from build123d import *

# Parameters (mm, degrees)
SKETCH3_W            = 2.76715
SKETCH3_H            = 2.76715
BOSS_EXTRUDE1_DEPTH  = 5
SKETCH4_W            = 2.76715
SKETCH4_H            = 2.76715
BOSS_EXTRUDE2_DEPTH  = 7.5
SKETCH5_W            = 2.76715
SKETCH5_H            = 2.76715
BOSS_EXTRUDE3_DEPTH  = 7.5
SKETCH6_W            = 2.76715
SKETCH6_H            = 2.76715
BOSS_EXTRUDE4_DEPTH  = 7.5
SKETCH7_W            = 2.76715
SKETCH7_H            = 2.76715
BOSS_EXTRUDE5_DEPTH  = 7.5
SKETCH8_W            = 2.76715
SKETCH8_H            = 2.76715
BOSS_EXTRUDE6_DEPTH  = 7.5
SKETCH9_W            = 2.76715
SKETCH9_H            = 2.76715
BOSS_EXTRUDE7_DEPTH  = 7.5
SKETCH10_W           = 2.76715
SKETCH10_H           = 2.76715
BOSS_EXTRUDE8_DEPTH  = 7.5
SKETCH11_W           = 2.76715
SKETCH11_H           = 2.76715
BOSS_EXTRUDE9_DEPTH  = 7.5
SKETCH12_W           = 2.76715
SKETCH12_H           = 2.76715
BOSS_EXTRUDE10_DEPTH = 7.5
SKETCH13_W           = 2.76715
SKETCH13_H           = 2.76715
BOSS_EXTRUDE11_DEPTH = 3.75
SKETCH14_W           = 2.76715
SKETCH14_H           = 2.76715
BOSS_EXTRUDE12_DEPTH = 10
SKETCH15_W           = 2.76715
SKETCH15_H           = 2.76715
BOSS_EXTRUDE13_DEPTH = 7.5
SKETCH16_W           = 2.76715
SKETCH16_H           = 2.76715
BOSS_EXTRUDE14_DEPTH = 3.75
SKETCH17_W           = 2.76715
SKETCH17_H           = 2.76715
BOSS_EXTRUDE15_DEPTH = 10
CUT_EXTRUDE3_START   = -0.5
CUT_EXTRUDE3_DEPTH   = 1.76715


with BuildPart() as part:
    # Sketch3 → Boss-Extrude1 (new, symmetric)
    with BuildSketch(Plane.XY):
        Rectangle(SKETCH3_W, SKETCH3_H)
    extrude(amount=BOSS_EXTRUDE1_DEPTH, both=True)

    # Sketch4 → Boss-Extrude2 (add)
    with BuildSketch(Plane(origin=(1.383575, 0, 0), x_dir=(0, 0, -1), z_dir=(1, 0, 0))):
        with Locations((-3.616425, 0)):
            Rectangle(SKETCH4_W, SKETCH4_H)
        with Locations((3.616425, 0)):
            Rectangle(SKETCH4_W, SKETCH4_H)
    extrude(amount=BOSS_EXTRUDE2_DEPTH)

    # Sketch5 → Boss-Extrude3 (add)
    with BuildSketch(Plane.XY.offset(5)):
        with Locations((7.5, 0)):
            Rectangle(SKETCH5_W, SKETCH5_H)
    extrude(amount=BOSS_EXTRUDE3_DEPTH)

    # Sketch6 → Boss-Extrude4 (add)
    with BuildSketch(Plane.ZY.offset(-6.116425)):
        with Locations((11.116425, 0)):
            Rectangle(SKETCH6_W, SKETCH6_H)
    extrude(amount=BOSS_EXTRUDE4_DEPTH)

    # Sketch7 → Boss-Extrude5 (add)
    with BuildSketch(Plane.XY.offset(12.5)):
        Rectangle(SKETCH7_W, SKETCH7_H)
    extrude(amount=BOSS_EXTRUDE5_DEPTH)

    # Sketch8 → Boss-Extrude6 (add)
    with BuildSketch(Plane(origin=(0, 0, -5), x_dir=(-1, 0, 0), z_dir=(0, 0, -1))):
        with Locations((-7.5, 0)):
            Rectangle(SKETCH8_W, SKETCH8_H)
    extrude(amount=BOSS_EXTRUDE6_DEPTH)

    # Sketch9 → Boss-Extrude7 (add)
    with BuildSketch(Plane.ZY.offset(-6.116425)):
        with Locations((-11.116425, 0)):
            Rectangle(SKETCH9_W, SKETCH9_H)
    extrude(amount=BOSS_EXTRUDE7_DEPTH)

    # Sketch10 → Boss-Extrude8 (add)
    with BuildSketch(Plane(origin=(0, 0, -12.5), x_dir=(-1, 0, 0), z_dir=(0, 0, -1))):
        Rectangle(SKETCH10_W, SKETCH10_H)
    extrude(amount=BOSS_EXTRUDE8_DEPTH)

    # Sketch11 → Boss-Extrude9 (add)
    with BuildSketch(Plane(origin=(1.383575, 0, 0), x_dir=(0, 0, -1), z_dir=(1, 0, 0))):
        with Locations((18.616425, 0)):
            Rectangle(SKETCH11_W, SKETCH11_H)
        with Locations((-18.616425, 0)):
            Rectangle(SKETCH11_W, SKETCH11_H)
    extrude(amount=BOSS_EXTRUDE9_DEPTH)

    # Sketch12 → Boss-Extrude10 (add)
    with BuildSketch(Plane(origin=(0, 0, -20), x_dir=(-1, 0, 0), z_dir=(0, 0, -1))):
        with Locations((-7.5, 0)):
            Rectangle(SKETCH12_W, SKETCH12_H)
    extrude(amount=BOSS_EXTRUDE10_DEPTH)

    # Sketch13 → Boss-Extrude11 (add)
    with BuildSketch(Plane.ZY.offset(-6.116425)):
        with Locations((-26.116425, 0)):
            Rectangle(SKETCH13_W, SKETCH13_H)
    extrude(amount=BOSS_EXTRUDE11_DEPTH)

    # Sketch14 → Boss-Extrude12 (add)
    with BuildSketch(Plane(origin=(0, 0, -27.5), x_dir=(-1, 0, 0), z_dir=(0, 0, -1))):
        with Locations((-3.75, 0)):
            Rectangle(SKETCH14_W, SKETCH14_H)
    extrude(amount=BOSS_EXTRUDE12_DEPTH)

    # Sketch15 → Boss-Extrude13 (add)
    with BuildSketch(Plane.XY.offset(20)):
        with Locations((7.5, 0)):
            Rectangle(SKETCH15_W, SKETCH15_H)
    extrude(amount=BOSS_EXTRUDE13_DEPTH)

    # Sketch16 → Boss-Extrude14 (add)
    with BuildSketch(Plane.ZY.offset(-6.116425)):
        with Locations((26.116425, 0)):
            Rectangle(SKETCH16_W, SKETCH16_H)
    extrude(amount=BOSS_EXTRUDE14_DEPTH)

    # Sketch17 → Boss-Extrude15 (add)
    with BuildSketch(Plane.XY.offset(27.5)):
        with Locations((3.75, 0)):
            Rectangle(SKETCH17_W, SKETCH17_H)
    extrude(amount=BOSS_EXTRUDE15_DEPTH)

    # Sketch23 → Cut-Extrude3 (cut)
    with BuildSketch(Plane(origin=(0, 1.383575, 0), x_dir=(1, 0, 0), z_dir=(0, 1, 0)).offset(CUT_EXTRUDE3_START)):
        Polygon((2.866425, 37.5), (4.633575, 37.5), (4.633575, 27), (8.383575, 27), (8.383575, 17.73285), (0.883575, 17.73285), (0.883575, 12), (8.383575, 12), (8.383575, 2.73285), (0.883575, 2.73285), (0.883575, -2.73285), (8.383575, -2.73285), (8.383575, -12), (0.883575, -12), (0.883575, -17.73285), (8.383575, -17.73285), (8.383575, -27), (4.633575, -27), (4.633575, -37.5), (2.866425, -37.5), (2.866425, -25.23285), (6.616425, -25.23285), (6.616425, -19.5), (-0.883575, -19.5), (-0.883575, -10.23285), (6.616425, -10.23285), (6.616425, -4.5), (-0.883575, -4.5), (-0.883575, 4.5), (6.616425, 4.5), (6.616425, 10.23285), (-0.883575, 10.23285), (-0.883575, 19.5), (6.616425, 19.5), (6.616425, 25.23285), (2.866425, 25.23285), align=None)
    extrude(amount=-CUT_EXTRUDE3_DEPTH, mode=Mode.SUBTRACT)


solid = part.part
The model under review builds one solid part; all positions refer to its coordinate system, in mm. A direction names the side the tool comes from. Coordinates: 2 decimals unless noted, no trailing zeros. Write each loop counter-clockwise with the first axis right and the second up, starting at its lowest first coordinate (ties: lowest second). Pieces come first, ordered by that corner, then holes. Notation, with made-up numbers: (-24.75, 34.5) - (1.25, 34.5) arc R21 cw to (1.25, 56.5) - close; hole circle Ø1 at (68, -12). An arc over 180 degrees is marked (long way). Answer as CSV lines item,"result".
(1) We need section B-B (z = -32). Give the boundary of the cut face in (x, y).
Data:
outline,"(2.37, -1.38) - (5.13, -1.38) - (5.13, 1.38) - (2.37, 1.38) - close; hole (2.87, -0.88) - (4.63, -0.88) - (4.63, 0.88) - (2.87, 0.88) - close"
(2) Mouldability with a two-part tool opening along X and no side actions: class faces 4 (the flat face through (-1.384, 0, 0)), 5 (the flat face through (-0.884, 0, -15)), 6 (the flat face through (5, 0, -17.233)) as pulls with the +X half, pulls with the -X half, needs draft (parallel to the pull), parting line crosses it, or undercut.
Data:
face 4,"pulls with the -X half"
face 5,"undercut"
face 6,"needs draft"
(3) We need section A-A (z = 18.5). Give the boundary of the cut face in (x, y).
Data:
outline,"(-1.38, -1.38) - (8.88, -1.38) - (8.88, 1.38) - (-1.38, 1.38) - close; hole (-0.88, -0.88) - (8.38, -0.88) - (8.38, 0.88) - (-0.88, 0.88) - close"
(4) Tool access review of faces 1 (the flat face through (8.384, 0, -22)), 2 (the flat face through (2.366, 0, -31)), 3 (the flat face through (4, 0, -24.733)): name each direction out of +Z, -Z, +X, -X, +Y, -Y from which nothing blocks a thin tool from reaching the whole face with its end or side.
Data:
face 1,"none"
face 2,"-Z, -X, +Y, -Y"
face 3,"-X, +Y, -Y"
(5) For line 1 along Z through (x, y) = (7.5, -1.05); line 2 along Y through (x, z) = (4.25, 10.5); line 3 along Z through (x, y) = (0.75, 0.1), list the stretches that pass through material, from the lowest coordinate up. Write a range as [from, to].
Data:
line 1,"z = [-27.5, -17.23], [-12.5, -2.23], [2.23, 12.5], [17.23, 27.5]"
line 2,"y = [-1.38, -0.88], [0.88, 1.38]"
line 3,"z = [-20, -19.5], [-10.23, -9.73], [-5, -4.5], [4.5, 5], [9.73, 10.23], [19.5, 20]"
(6) Clearance check with flat-ended pins moving along their axes: pin 1 Ø0.8 at (y, z) = (0, -14) entering from +X; pin 2 Ø0.5 at (x, y) = (1.5, 0) entering from +Z; pin 3 Ø1.5 at (x, y) = (7.5, -0.5) entering from +Z. State where each tip first meets the part, or that it passes through.
Data:
pin 1,"stops at x = 1.38"
pin 2,"stops at z = 20"
pin 3,"stops at z = 27.5"
